from build123d import *

# Parameters (mm, degrees)
SKETCH6_W          = 55.097235346
SKETCH6_H          = 50
MAIN_BODY_DEPTH    = 13
MAIN_HOLE_DEPTH    = 56.097235346
EXTERIOR_FILLET_R  = 3
SKETCH9_R          = 3.3
BOLT_HOLES_DEPTH   = 14
TOP_HOLE_FILLET_R  = 5
SIDE_HOLE_FILLET_R = 4


with BuildPart() as part:
    # Sketch6 → Main Body (new body)
    with BuildSketch(Plane(origin=(0, 68, 0), x_dir=(1, 0, 0), z_dir=(0, 1, 0))):
        with Locations((-0.048617673, 0)):
            Rectangle(SKETCH6_W, SKETCH6_H)
    extrude(amount=MAIN_BODY_DEPTH)

    # Sketch7 → Main Hole (cut, through all)
    with BuildSketch(Plane(origin=(27.5, 0, 0), x_dir=(0, 0, -1), z_dir=(1, 0, 0))):
        Polygon((0, 74.5), (-9.282962044, 68), (0, 61.5), (9.282962044, 68), align=None)
    extrude(amount=-MAIN_HOLE_DEPTH, mode=Mode.SUBTRACT)

    # Exterior Fillet
    exterior_fillet_edges = [part.edges().sort_by_distance(p)[0] for p in [
        (-27.597235346, 74.5, 25),
        (-27.597235346, 74.5, -25),
    ]]
    fillet(exterior_fillet_edges, radius=EXTERIOR_FILLET_R)

    # Sketch9 → Bolt Holes (cut, through all)
    with BuildSketch(Plane(origin=(0, 81, 0), x_dir=(1, 0, 0), z_dir=(0, 1, 0))):
        with Locations((15.473743703, -17.201232435)):
            Circle(SKETCH9_R)
        with Locations((-11, -17.201232435)):
            Circle(SKETCH9_R)
        with Locations((15.473743703, 17.324336932)):
            Circle(SKETCH9_R)
        with Locations((-11, 17.324336932)):
            Circle(SKETCH9_R)
    extrude(amount=-BOLT_HOLES_DEPTH, mode=Mode.SUBTRACT)

    # Top Hole Fillet
    top_hole_fillet_edges = [part.edges().sort_by_distance(p)[0] for p in [
        (-0.048617673, 74.5, 0),
    ]]
    fillet(top_hole_fillet_edges, radius=TOP_HOLE_FILLET_R)

    # Side Hole Fillet
    side_hole_fillet_edges = [part.edges().sort_by_distance(p)[0] for p in [
        (-0.048617673, 68, -9.282962044),
        (-0.048617673, 68, 9.282962044),
    ]]
    fillet(side_hole_fillet_edges, radius=SIDE_HOLE_FILLET_R)


solid = part.part
Design review of the part built by this model. Coordinates are the model's own, in mm. A direction names the side the tool comes from. Coordinates: 2 decimals unless noted, no trailing zeros. Write each loop counter-clockwise with the first axis right and the second up, starting at its lowest first coordinate (ties: lowest second). Pieces come first, ordered by that corner, then holes. Notation, with made-up numbers: (51, -39.75) - (80, -39.75) arc R27 ccw to (80, -0.75) - close; hole circle Ø11 at (-27.5, 45). An arc over 180 degrees is marked (long way). One line per item, written item: value.
1) For faces 1 (the face through (0, 68, 18)), 2 (the face through (-0.4, 68.2, -9.3)), list the 3-axis set-ups (+Z, -Z, +X, -X, +Y, -Y) from which the entire face can be reached by the end or side of a thin tool; tool diameter is ignored.
Answer sheet:
face 1: +Z, -Z, +X, -X, -Y
face 2: +X, -X, -Y
2) To check wall thickness, follow probe 1 along X at (y, z) = (80.25, 17); probe 2 along Z at (x, y) = (-11, 74.5); probe 3 along Z at (x, y) = (-8, 70.5). State the ranges of each line that lie inside material, in increasing order.
Answer sheet:
probe 1: x = -27.6 to -14.29, -7.71 to 12.18, 18.77 to 27.5
probe 2: z = -25 to -20.62, -14.02 to 13.9, 20.5 to 25
probe 3: z = -25 to -18.7, -15.95 to -5.71, 5.71 to 15.83, 18.58 to 25
3) Mouldability with a two-part tool opening along Z and no side actions: class faces 3 (the face through (-27.597, 74, 0)), 4 (the face through (1, 74, 25)), 5 (the face through (0.34, 70.58, -5.6)) as +Z half, -Z half, draft (parallel to the pull), parting line (faces both ways), or undercut.
Answer sheet:
face 3: draft
face 4: +Z half
face 5: undercut
4) Insertion check: pin 1 (12 mm diameter, centred on x = 16, z = 2.5, fed in from -Y); pin 2 (4 mm diameter, centred on x = -1, z = 2, fed in from -Y); pin 3 (6 mm diameter, centred on x = 15.47, z = -17.32, fed in from +Y); pin 4 (5 mm diameter, centred on x = 10, z = 3.5, fed in from -Y). Each pin has a flat end and moves straight along its axis. Give the tip position at first contact, or say it passes through.
Answer sheet:
pin 1: stops at y = 68.56
pin 2: stops at y = 71.7
pin 3: passes through
pin 4: stops at y = 70.3
5) Add section B-B (y = 71). State the section outline as (x, z) points, plus the area to 3 significant figures.
Answer sheet:
outline: (-27.6, -22) arc R3 ccw to (-24.6, -25) - (27.5, -25) - (27.5, -5) - (-27.6, -5) - close; (-27.6, 5) - (27.5, 5) - (27.5, 25) - (-24.6, 25) arc R3 ccw to (-27.6, 22) - close; hole circle Ø6.6 at (-11, -17.32); hole circle Ø6.6 at (-11, 17.2); hole circle Ø6.6 at (15.47, -17.32); hole circle Ø6.6 at (15.47, 17.2)
area: 2,060 mm2
6) Add section C-C (x = -20). State the section outline as (y, z) points.
Answer sheet:
outline: (68, -25) - (81, -25) - (81, 25) - (68, 25) - (68, 10.54) arc R4 ccw to (68.72, 8.25) - (72.49, 2.87) arc R5 cw to (72.49, -2.87) - (68.72, -8.25) arc R4 ccw to (68, -10.54) - close
7) Add section A-A (x = -11). State the section outline as (y, z) points.
Answer sheet:
outline: (68, -25) - (81, -25) - (81, -20.62) - (68, -20.62) - close; (68, -14.02) - (81, -14.02) - (81, 13.9) - (68, 13.9) - (68, 10.54) arc R4 ccw to (68.72, 8.25) - (72.49, 2.87) arc R5 cw to (72.49, -2.87) - (68.72, -8.25) arc R4 ccw to (68, -10.54) - close; (68, 20.5) - (81, 20.5) - (81, 25) - (68, 25) - close
8) Add section D-D (y = 74.75). State the section outline as (x, z) points.
Answer sheet:
outline: (-27.6, -22) arc R3 ccw to (-24.6, -25) - (27.5, -25) - (27.5, 25) - (-24.6, 25) arc R3 ccw to (-27.6, 22) - close; hole circle Ø6.6 at (-11, -17.32); hole circle Ø6.6 at (-11, 17.2); hole circle Ø6.6 at (15.47, -17.32); hole circle Ø6.6 at (15.47, 17.2)
